Verification items for this drawing (mm, ordinates from the low corner). Round coordinates to 2 decimals unless told otherwise and drop trailing zeros. Order: outer loops, then holes, each group sorted by start corner. A loop starts at its lowest first (then second) coordinate and runs counter-clockwise, first axis right, second up. Notation, with made-up numbers: (-2, 85.5) -> (37, 85.5) arc R19 cw to (37, 102.5) -> close; hole circle Ø2 at (-22.5, 0.25). An arc over 180 degrees is marked (long way). Put each result on its own line as item: value.
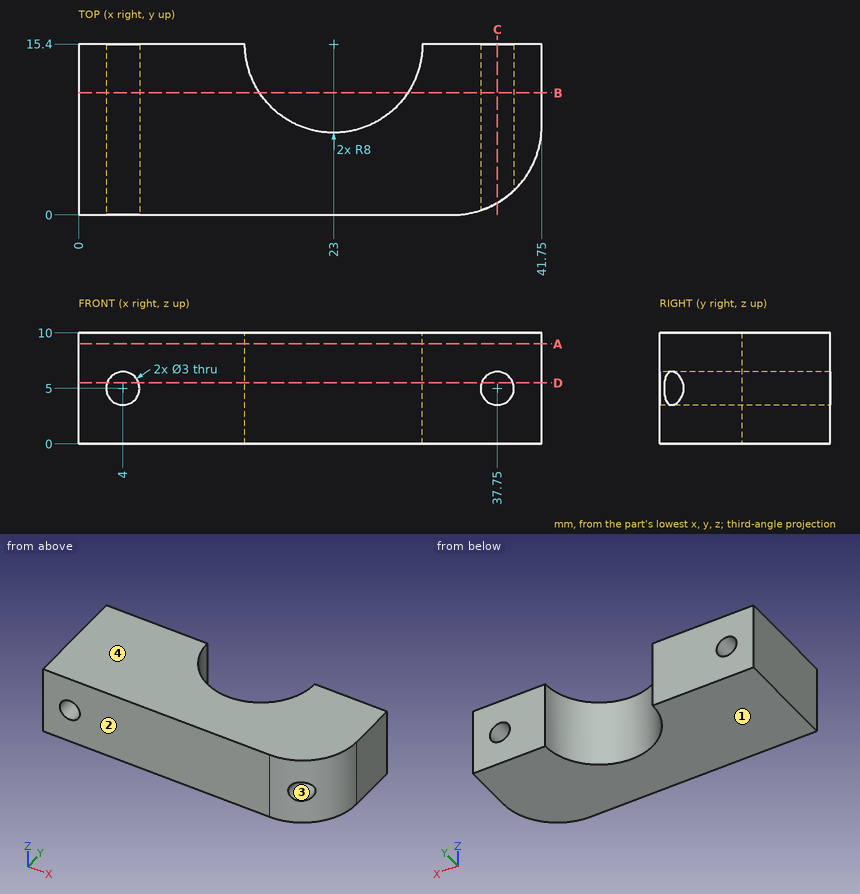
Item 1: Material ranges on L1, parallel to X at y = 9.25, z = 5; L2, parallel to X at y = 11.25, z = 4.5; L3, parallel to Z at x = 37.75, y = 8, recorded low to high. Write a range as [from, to].
Check sheet entries:
L1: x = [0, 2.5], [5.5, 17.88], [28.12, 36.25], [39.25, 41.75]
L2: x = [0, 2.59], [5.41, 16.16], [29.84, 36.34], [39.16, 41.75]
L3: z = [0, 3.5], [6.5, 10]
Item 2: Section check C-C on x = 37.75. Record the boundary of the cut face in (y, z), then the cut area to 3 significant figures.
Check sheet entries:
outline: (1.07, 0) -> (15.4, 0) -> (15.4, 3.5) -> (1.07, 3.5) -> close; (1.07, 6.5) -> (15.4, 6.5) -> (15.4, 10) -> (1.07, 10) -> close
area: 100 mm^2
Item 3: Section check B-B on y = 11. Record the boundary of the cut face in (x, z), then the cut area to 3 significant figures.
Check sheet entries:
outline: (0, 0) -> (16.32, 0) -> (16.32, 10) -> (0, 10) -> close; (29.68, 0) -> (41.75, 0) -> (41.75, 10) -> (29.68, 10) -> close; hole circle Ø3 at (4, 5); hole circle Ø3 at (37.75, 5)
area: 270 mm^2
Item 4: Gauge pin test, flat end, axial feed: pin 1 Ø2 at (y, z) = (2, 5.5) entering from +X (3 decimals). Record the tip position at first contact, or that the pin passes through.
Check sheet entries:
pin 1: stops at x = 39.995
Item 5: Release check for a two-part mould opening along Z. For the marked faces 1, 2, 3 and 4 record: +Z half, -Z half, draft (parallel to the pull), parting line (faces both ways), or undercut.
Check sheet entries:
face 1: -Z half
face 2: draft
face 3: undercut
face 4: +Z half
Item 6: Section check D-D on z = 5.5. Record the boundary of the cut face in (x, y).
Check sheet entries:
outline: (0, 0) -> (2.59, 0) -> (2.59, 15.4) -> (0, 15.4) -> close; (5.41, 0) -> (33.75, 0) arc R8 ccw to (36.34, 0.43) -> (36.34, 15.4) -> (31, 15.4) arc R8 cw to (15, 15.4) -> (5.41, 15.4) -> close; (39.16, 2.11) arc R8 ccw to (41.75, 8) -> (41.75, 15.4) -> (39.16, 15.4) -> close
Item 7: Section check A-A on z = 9. Record the boundary of the cut face in (x, y).
Check sheet entries:
outline: (0, 0) -> (33.75, 0) arc R8 ccw to (41.75, 8) -> (41.75, 15.4) -> (31, 15.4) arc R8 cw to (15, 15.4) -> (0, 15.4) -> close
